Can you work these out from the drawing? Everything is in mm from the part's minimum corner. A direction names the side the tool comes from. Round coordinates to 2 decimals unless told otherwise and drop trailing zeros. Order: outer loops, then holes, each group sorted by start corner. A loop starts at its lowest first (then second) coordinate and runs counter-clockwise, first axis right, second up. Notation, with made-up numbers: (73.5, -25) -> (102.5, -25) arc R27 cw to (102.5, 6) -> close; hole circle Ø4 at (-19, 15). An arc over 180 degrees is marked (long way). One line per item, written item: value.
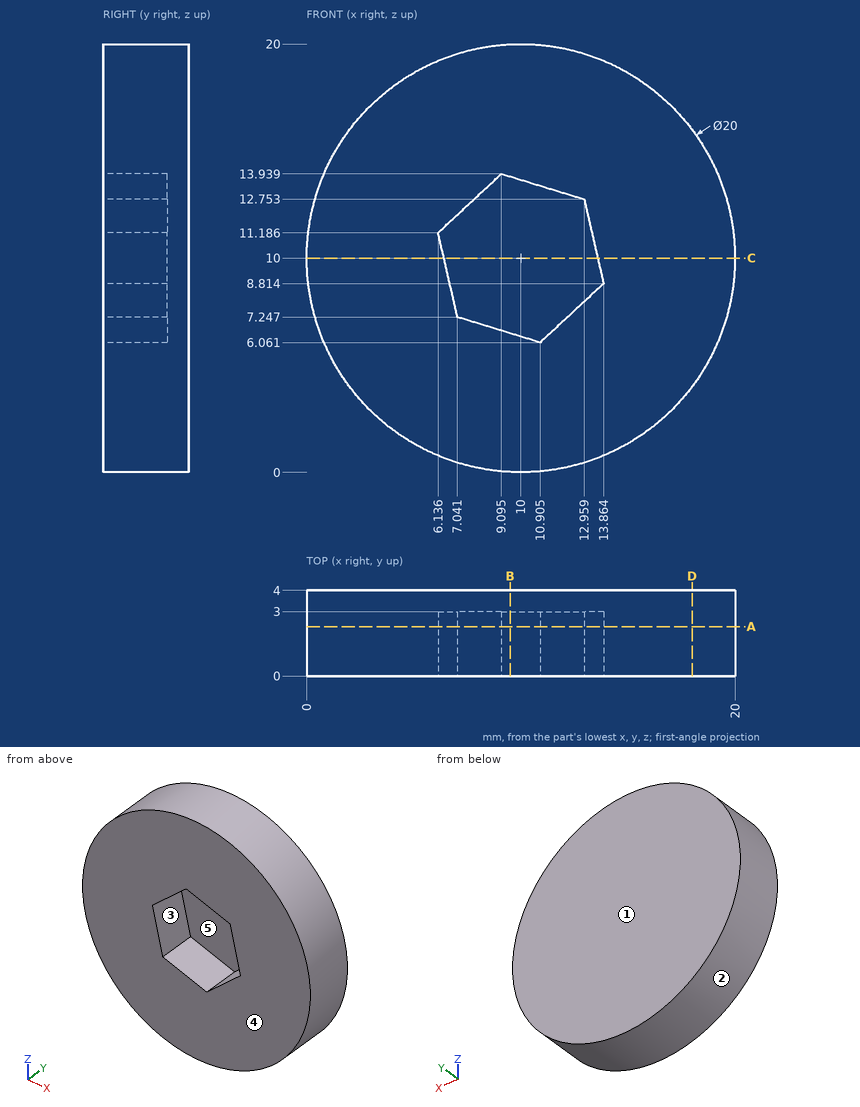
Q1. Please list where these lines run through material, in increasing order: line 1 along Z through (x, y) = (10.5, 2.6) (1 decimal); line 2 along Z through (x, y) = (8, 0.8) (1 decimal); line 3 along Y through (x, z) = (9.25, 9.75).
Answers below:
line 1: 0 to 6.2, 13.5 to 20
line 2: 0.2 to 7, 12.9 to 19.8
line 3: 3 to 4
Q2. Will these pins go through, and if not, where does the flat tip stop? pin 1 Ø1 at (x, y) = (7, 1.5) entering from -Z; pin 2 Ø1.5 at (x, y) = (17, 0.5) entering from +Z (1 decimal).
Answers below:
pin 1: z = 0.32
pin 2: z = 17.8
Q3. I want a section at B-B on x = 9.5. List the corners of the cut face in (y, z) for me (1 decimal).
Answers below:
outline: (0, 0) -> (4, 0) -> (4, 20) -> (0, 20) -> (0, 13.8) -> (3, 13.8) -> (3, 6.5) -> (0, 6.5) -> close
Q4. I want a section at A-A on y = 2.3. List the corners of the cut face in (x, z) for me (1 decimal).
Answers below:
outline: circle Ø20 at (10, 10); hole (6.1, 11.2) -> (7, 7.2) -> (10.9, 6.1) -> (13.9, 8.8) -> (13, 12.8) -> (9.1, 13.9) -> close
Q5. We'd pull the mould along Z, two halves only. Please class the marked faces 1, 2 and 3: released by +Z, released by -Z, zero draft, split by the parting line, or undercut.
Answers below:
face 1: zero draft
face 2: split by the parting line
face 3: undercut
Q6. I want a section at D-D on x = 18. List the corners of the cut face in (y, z) for me, plus the area to 3 significant figures.
Answers below:
outline: (0, 4) -> (4, 4) -> (4, 16) -> (0, 16) -> close
area: 48.0 mm^2
Q7. On a 3-axis mill with a long thin cutter (end or side, diameter ignored), from which of +Z, -Z, +X, -X, +Y, -Y can I reach the whole of each face in a straight line? I mean the marked faces 4 and 5. Say none if no direction works.
Answers below:
face 4: +Z, -Z, +X, -X, -Y
face 5: -Y
Q8. I want a section at C-C on z = 10. List the corners of the cut face in (x, y) for me.
Answers below:
outline: (0, 0) -> (6.41, 0) -> (6.41, 3) -> (13.59, 3) -> (13.59, 0) -> (20, 0) -> (20, 4) -> (0, 4) -> close
